Can you work these out from the model? Positions are in its coordinate system, mm. A direction names the side the tool comes from. Give positions to 0.01 mm unless a question says otherwise; leave off trailing zeros. Loops run counter-clockwise (first coordinate to the right, second up) from the corner with the lowest first, then second, coordinate; pieces in that order, holes last. Notation, with made-up numbers: (50.25, 10) - (74.25, 10) arc R22 ccw to (74.25, 24) - close; hole circle Ø11 at (39.25, 72.5). An arc over 180 degrees is marked (long way). Answer in a Markdown table with one row per item.
Autodesk Inventor part; units mm, degrees
ref_plane "YZ Plane" through (0, 0, 0) normal (1, 0, 0) x (0, 1, 0)
ref_plane "XZ Plane" through (0, 0, 0) normal (0, 1, 0) x (-1, 0, 0)
ref_plane "XY Plane" through (0, 0, 0) normal (0, 0, 1) x (1, 0, 0)
sketch "Sketch1" plane through (0, 0, 0) normal (0, 1, 0) x (-1, 0, 0)
  line L0 (37, 37) -> (-37, 37)
  line L1 (-37, 37) -> (-37, -37)
  line L2 (-37, -37) -> (37, -37)
  line L3 (37, -37) -> (37, 37)
  point P0 (0, 0)
  dimension "d0" = 74
  dimension "d1" = 74
extrude "Extrusion1" add sketch "Sketch1" along normal blind 6
fillet "Fillet1" radius 5 4 edges at (-37, 3, 37) (37, 3, 37) (37, 3, -37) (-37, 3, -37)
sketch "Sketch2" plane through (0, 6, 0) normal (0, 1, 0) x (1, 0, 0)
  line L0 (-37, 32) -> (-37, -32)
  line L1 (-37, 0) -> (37, 0)
  line L2 (37, -32) -> (37, 32)
  circle A0 centre (0, 0) radius 6
  line L3 (-37, 0) -> (37, 0)
  line L4 (37, 0) -> (37, 63.5)
  line L5 (37, 63.5) -> (-37, 63.5)
  line L6 (-37, 63.5) -> (-37, 0)
  line L7 (-6, 0) -> (-26, 0)
  line L8 (-26, 0) -> (-37, 11)
  line L9 (6, 0) -> (26, 0)
  line L10 (26, 0) -> (37, 11)
  circle A1 centre (32, 0) radius 2
  circle A2 centre (0, -32) radius 2
  circle A3 centre (-32, 0) radius 2
  point P0 (-6, 0)
  dimension "d5" = 12
  dimension "d6" = 20
  dimension "d7" = 135
  dimension "d8" = 20
  dimension "d9" = 135
  dimension "d10" = 4
  dimension "d11" = 4
  dimension "d12" = 4
extrude "Extrusion2" cut sketch "Sketch2" against normal blind 10 contours L6 L5 L4 L2 L10 L1 A0 L8 L0 | A3 L1 | L1 A3 | A0 L1 | L1 A0 | A1 L1 | L1 A1 | A2
sketch "Sketch3" plane through (0, 6, 0) normal (0, 1, 0) x (1, 0, 0)
  line L0 (11, -5) -> (17, -5)
  line L1 (17, -5) -> (17, -25)
  line L2 (17, -25) -> (11, -25)
  line L3 (11, -25) -> (11, -5)
  line L4 (-11, -5) -> (-17, -5)
  line L5 (-17, -5) -> (-17, -25)
  line L6 (-17, -25) -> (-11, -25)
  line L7 (-11, -25) -> (-11, -5)
  point P0 (0, 0)
  dimension "d15" = 6
  dimension "d16" = 20
  dimension "d17" = 6
extrude "Extrusion3" cut sketch "Sketch3" against normal blind 10
sketch "Sketch4" plane through (26, 6, 0) normal (0, 0, -1) x (-1, 0, 0)
  circle A0 centre (12, -3) radius 2
  circle A1 centre (40, -3) radius 2
  point P0 (26, -6)
  dimension "d20" = 4
  dimension "d21" = 4
extrude "Extrusion4" cut sketch "Sketch4" against normal blind 10
fillet "Fillet2" radius 2 5 edges at (35.5355, 6, 35.5355) (0, 6, 37) (-35.5355, 6, 35.5355) (-37, 6, 10.5) (37, 6, 10.5)
sketch "Sketch5" plane through (0, 6, 0) normal (0, 1, 0) x (1, 0, 0)
  circle A0 centre (23, -7) radius 2
  circle A1 centre (-23, -7) radius 2
  point P0 (0, 0)
  dimension "d25" = 4
  dimension "d26" = 4
extrude "Extrusion5" cut sketch "Sketch5" against normal blind 10
properties part number "g2HEMount1"
Q1. Imagine slicing it at D-D, the plane y = 1.8. Count the separate pieces of the cut face and the enclosed holes in it, and give its area (3 significant figures).
Checked values:
| item | result |
|---|---|
| separate pieces | 1 |
| enclosed holes | 5 |
| area | 2,460 mm² |
Q2. Imagine slicing it at C-C, the plane x = 14. Write out the boundary of the cut face in (y, z).
Checked values:
| item | result |
|---|---|
| outline | (0, 0) - (1, 0) - (1, 5) - (0, 5) - close; (0, 25) - (6, 25) - (6, 35) arc R2 ccw to (4, 37) - (0, 37) - close; (5, 0) - (6, 0) - (6, 5) - (5, 5) - close |
Q3. For pin 1 (3.5 mm diameter, centred on x = 14, y = 3, fed in from -Z); pin 2 (3 mm diameter, centred on x = 14, y = 4, fed in from -Z), each with a flat end and sliding along its axis, tell me the tip position at first contact or that it passes through.
Checked values:
| item | result |
|---|---|
| pin 1 | stops at z = 25 |
| pin 2 | stops at z = 0 |
Q4. Imagine slicing it at B-B, the plane x = 23. Write out the boundary of the cut face in (y, z), and give its area (3 significant figures).
Checked values:
| item | result |
|---|---|
| outline | (0, 0) - (6, 0) - (6, 5) - (0, 5) - close; (0, 9) - (6, 9) - (6, 35) arc R2 ccw to (4, 37) - (0, 37) - close |
| area | 197 mm² |
Q5. On a 3-axis mill with a long thin cutter (end or side, diameter ignored), from which of +Z, -Z, +X, -X, +Y, -Y can I reach the whole of each face in a straight line? I mean faces 1 (the face through (-13, 5, 5)), 2 (the face through (-16, 4, 0)), 3 (the face through (-37, 2, 10)). Say none if no direction works.
Checked values:
| item | result |
|---|---|
| face 1 | +Y, -Y |
| face 2 | -Z, +Y, -Y |
| face 3 | +Z, -Z, -X, +Y, -Y |
Q6. If I drill on line 1 (X direction, y = 3.9, z = 7); line 2 (X direction, y = 2.5, z = 20.5); line 3 (Z direction, x = 0, y = 3.1), over which ranges is the centre line in solid material (lowest first)? Write a range as [from, to].
Checked values:
| item | result |
|---|---|
| line 1 | x = [-37, -25], [-21, -17], [-11, 11], [17, 21], [25, 37] |
| line 2 | x = [-37, -17], [-11, 11], [17, 37] |
| line 3 | z = [6, 30], [34, 37] |
Q7. If we mould it in two halves opening along X, with no side actions, what happens to faces 4 (the face through (35, 2, 36)), 5 (the face through (33.847, 3.042, 0.766)), 6 (the face through (-36.43, 5.4, 10.2))? For each: released by +X, released by -X, zero draft, split by the parting line, or undercut.
Checked values:
| item | result |
|---|---|
| face 4 | released by +X |
| face 5 | undercut |
| face 6 | released by -X |
Q8. Imagine slicing it at A-A, the plane z = -5. Write out the boundary of the cut face in (x, y), and give its area (3 significant figures).
Checked values:
| item | result |
|---|---|
| outline | (-37, 0) - (-31, 0) - (-31, 6) - (-35, 6) arc R2 ccw to (-37, 4) - close; (31, 0) - (37, 0) - (37, 4) arc R2 ccw to (35, 6) - (31, 6) - close |
| area | 70.3 mm² |
